Check sheet for the drawn part. Datum: minimum x, y, z corner. Units: mm. A direction names the side the tool comes from. Round coordinates to 2 decimals unless told otherwise and drop trailing zeros. Loops run counter-clockwise (first coordinate to the right, second up) from the corner with the lowest first, then second, coordinate; pieces in that order, holes last.
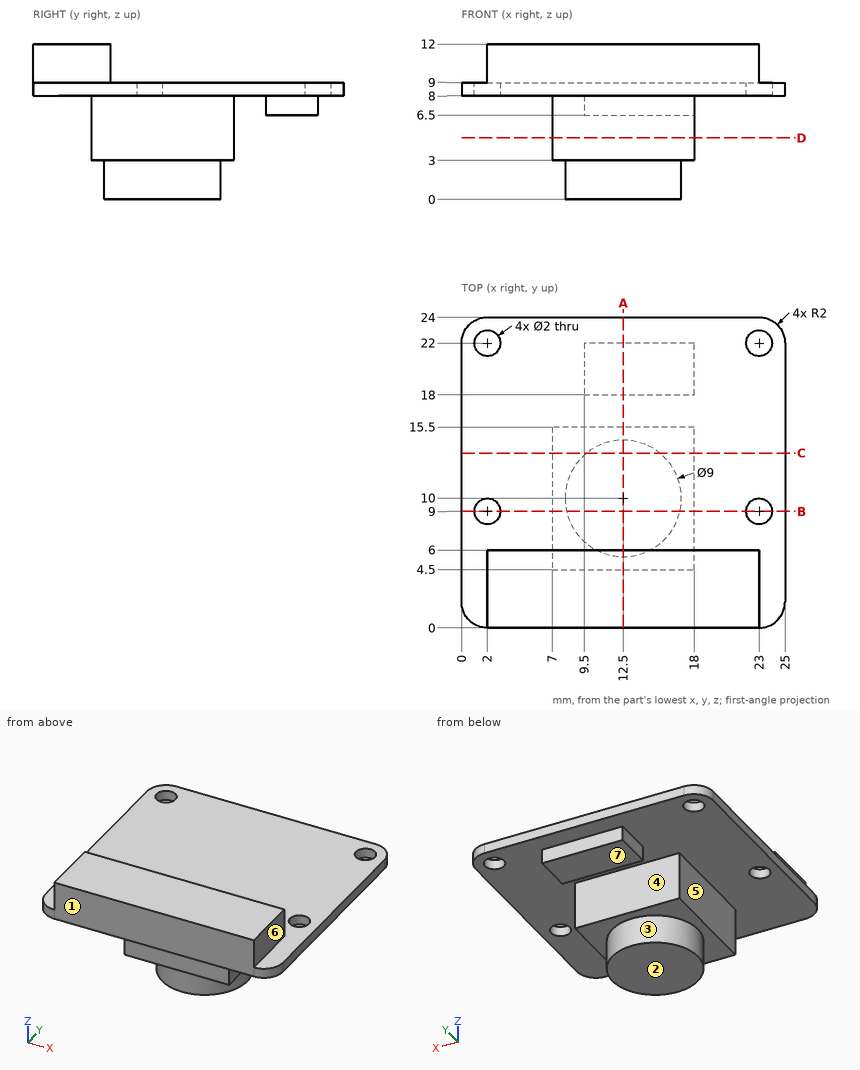
1) Sectioned sample at D-D, the plane z = 4.75. Record the cut outline in (x, y).
Report:
outline: (7, 4.5) - (18, 4.5) - (18, 15.5) - (7, 15.5) - close
2) Sectioned sample at B-B, the plane y = 9. Record the cut outline in (x, z).
Report:
outline: (0, 8) - (1, 8) - (1, 9) - (0, 9) - close; (3, 8) - (7, 8) - (7, 3) - (8.11, 3) - (8.11, 0) - (16.89, 0) - (16.89, 3) - (18, 3) - (18, 8) - (22, 8) - (22, 9) - (3, 9) - close; (24, 8) - (25, 8) - (25, 9) - (24, 9) - close
3) Sectioned sample at C-C, the plane y = 13.5. Record the cut outline in (x, z), then the cut area to 3 significant figures.
Report:
outline: (0, 8) - (7, 8) - (7, 3) - (9.67, 3) - (9.67, 0) - (15.33, 0) - (15.33, 3) - (18, 3) - (18, 8) - (25, 8) - (25, 9) - (0, 9) - close
area: 97.0 mm2
4) Gauge pin test, flat ends, axial feed: pin 1 (2.5 mm diameter, centred on x = 10.5, z = 6, fed in from -Y); pin 2 (1.5 mm diameter, centred on x = 12, z = 4.5, fed in from +Y); pin 3 (5 mm diameter, centred on x = 9.5, y = 21, fed in from +Z); pin 4 (1.5 mm diameter, centred on y = 3.5, z = 6, fed in from -X). Record the tip position at first contact, or that the pin passes through.
Report:
pin 1: stops at y = 4.5
pin 2: stops at y = 15.5
pin 3: stops at z = 9
pin 4: passes through
5) Sectioned sample at A-A, the plane x = 12.5. Record the cut outline in (y, z).
Report:
outline: (0, 8) - (4.5, 8) - (4.5, 3) - (5.5, 3) - (5.5, 0) - (14.5, 0) - (14.5, 3) - (15.5, 3) - (15.5, 8) - (18, 8) - (18, 6.5) - (22, 6.5) - (22, 8) - (24, 8) - (24, 9) - (6, 9) - (6, 12) - (0, 12) - close
6) Mould release check, pull along Y, two halves, no side actions. Record for the marked faces 1, 2, 3 and 4: +Y half, -Y half, draft (parallel to the pull), parting line (faces both ways), or undercut.
Report:
face 1: -Y half
face 2: draft
face 3: parting line
face 4: undercut
7) Access from +Z, -Z, +X, -X, +Y, -Y to the whole of each face (thin tool, end or side, straight path). Record for the marked faces 5, 6 and 7.
Report:
face 5: -Z, -X, +Y, -Y
face 6: +Z, +X, +Y, -Y
face 7: -Z, +X, -X, +Y
8) Scan lines: line 1 along Y through (x, z) = (23, 8.8); line 2 along X through (y, z) = (15, 5); line 3 along Z through (x, y) = (1.5, 17.5). Record each from-to range of solid material in increasing order.
Report:
line 1: y = 0 to 8, 10 to 21, 23 to 24
line 2: x = 7 to 18
line 3: z = 8 to 9
